from build123d import *

# Parameters (mm, degrees)
BOSS_EXTRUDE1_DEPTH = 64.25


with BuildPart() as part:
    # Sketch1 → Boss-Extrude1 (new body, symmetric)
    with BuildSketch(Plane(origin=(0, 0, 0), x_dir=(1, 0, 0), z_dir=(0, 1, 0))):
        with BuildLine():
            Line((-27.932619, -6.859853), (-27.932619, 5.140147))
            ThreePointArc((-27.932619, 5.140147), (-26.761046, 7.968574), (-23.932619, 9.140147))
            Line((-23.932619, 9.140147), (-11.932619, 9.140147))
            Line((-11.932619, 9.140147), (-11.932619, 4.640147))
            Line((-11.932619, 4.640147), (-19.182619, 4.640147))
            Line((-19.182619, 4.640147), (-19.182619, 3.140147))
            Line((-19.182619, 3.140147), (-12.932619, -3.109853))
            Line((-12.932619, -3.109853), (-7.932619, -3.109853))
            Line((-7.932619, -3.109853), (-2.932619, -3.109853))
            Line((-2.932619, -3.109853), (3.317381, 3.140147))
            Line((3.317381, 3.140147), (3.317381, 4.640147))
            Line((3.317381, 4.640147), (-3.932619, 4.640147))
            Line((-3.932619, 4.640147), (-3.932619, 9.140147))
            Line((-3.932619, 9.140147), (8.067381, 9.140147))
            ThreePointArc((8.067381, 9.140147), (10.895808, 7.968574), (12.067381, 5.140147))
            Line((12.067381, 5.140147), (12.067381, -6.859853))
            Line((12.067381, -6.859853), (7.567381, -6.859853))
            Line((7.567381, -6.859853), (7.567381, 0.390147))
            Line((7.567381, 0.390147), (6.067381, 0.390147))
            Line((6.067381, 0.390147), (-0.182619, -5.859853))
            Line((-0.182619, -5.859853), (-0.182619, -10.859853))
            Line((-0.182619, -10.859853), (-0.182619, -15.859853))
            Line((-0.182619, -15.859853), (6.067381, -22.109853))
            Line((6.067381, -22.109853), (7.567381, -22.109853))
            Line((7.567381, -22.109853), (7.567381, -14.859853))
            Line((7.567381, -14.859853), (12.067381, -14.859853))
            Line((12.067381, -14.859853), (12.067381, -26.859853))
            ThreePointArc((12.067381, -26.859853), (10.895808, -29.68828), (8.067381, -30.859853))
            Line((8.067381, -30.859853), (-3.932619, -30.859853))
            Line((-3.932619, -30.859853), (-3.932619, -26.359853))
            Line((-3.932619, -26.359853), (3.317381, -26.359853))
            Line((3.317381, -26.359853), (3.317381, -24.859853))
            Line((3.317381, -24.859853), (-2.932619, -18.609853))
            Line((-2.932619, -18.609853), (-7.932619, -18.609853))
            Line((-7.932619, -18.609853), (-12.932619, -18.609853))
            Line((-12.932619, -18.609853), (-19.182619, -24.859853))
            Line((-19.182619, -24.859853), (-19.182619, -26.359853))
            Line((-19.182619, -26.359853), (-11.932619, -26.359853))
            Line((-11.932619, -26.359853), (-11.932619, -30.859853))
            Line((-11.932619, -30.859853), (-23.932619, -30.859853))
            ThreePointArc((-23.932619, -30.859853), (-26.761046, -29.68828), (-27.932619, -26.859853))
            Line((-27.932619, -26.859853), (-27.932619, -14.859853))
            Line((-27.932619, -14.859853), (-23.432619, -14.859853))
            Line((-23.432619, -14.859853), (-23.432619, -22.109853))
            Line((-23.432619, -22.109853), (-21.932619, -22.109853))
            Line((-21.932619, -22.109853), (-15.682619, -15.859853))
            Line((-15.682619, -15.859853), (-15.682619, -10.859853))
            Line((-15.682619, -10.859853), (-15.682619, -5.859853))
            Line((-15.682619, -5.859853), (-21.932619, 0.390147))
            Line((-21.932619, 0.390147), (-23.432619, 0.390147))
            Line((-23.432619, 0.390147), (-23.432619, -6.859853))
            Line((-23.432619, -6.859853), (-27.932619, -6.859853))
        make_face()
        with BuildLine():
            Line((-25.932619, 2.390147), (-25.932619, 5.140147))
            ThreePointArc((-25.932619, 5.140147), (-25.346832, 6.554361), (-23.932619, 7.140147))
            Line((-23.932619, 7.140147), (-21.182619, 7.140147))
            Line((-21.182619, 7.140147), (-21.182619, 3.097254))
            Line((-21.182619, 3.097254), (-20.734396, 2.649031))
            Line((-20.734396, 2.649031), (-21.441502, 1.941924))
            Line((-21.441502, 1.941924), (-21.889726, 2.390147))
            Line((-21.889726, 2.390147), (-25.932619, 2.390147))
        make_face(mode=Mode.SUBTRACT)
        with BuildLine():
            Line((-20.380842, 0.881264), (-13.682619, -5.816959))
            Line((-13.682619, -5.816959), (-13.682619, -7.955115))
            Line((-13.682619, -7.955115), (-13.182619, -7.955115))
            Line((-13.182619, -7.955115), (-12.002324, -7.955115))
            ThreePointArc((-12.002324, -7.955115), (-11.468153, -7.324319), (-10.837356, -6.790148))
            Line((-10.837356, -6.790148), (-10.837356, -5.609853))
            Line((-10.837356, -5.609853), (-10.837356, -5.109853))
            Line((-10.837356, -5.109853), (-12.975512, -5.109853))
            Line((-12.975512, -5.109853), (-19.673735, 1.588371))
            Line((-19.673735, 1.588371), (-20.380842, 0.881264))
        make_face(mode=Mode.SUBTRACT)
        with BuildLine():
            Line((10.067381, 2.390147), (10.067381, 5.140147))
            ThreePointArc((10.067381, 5.140147), (9.481595, 6.554361), (8.067381, 7.140147))
            Line((8.067381, 7.140147), (5.317381, 7.140147))
            Line((5.317381, 7.140147), (5.317381, 3.097254))
            Line((5.317381, 3.097254), (4.869158, 2.649031))
            Line((4.869158, 2.649031), (5.576265, 1.941924))
            Line((5.576265, 1.941924), (6.024488, 2.390147))
            Line((6.024488, 2.390147), (10.067381, 2.390147))
        make_face(mode=Mode.SUBTRACT)
        with BuildLine():
            Line((-2.182619, -5.816959), (-2.182619, -7.955115))
            Line((-2.182619, -7.955115), (-2.682619, -7.955115))
            Line((-2.682619, -7.955115), (-3.862914, -7.955115))
            ThreePointArc((-3.862914, -7.955115), (-4.397085, -7.324319), (-5.027881, -6.790148))
            Line((-5.027881, -6.790148), (-5.027881, -5.609853))
            Line((-5.027881, -5.609853), (-5.027881, -5.109853))
            Line((-5.027881, -5.109853), (-2.889726, -5.109853))
            Line((-2.889726, -5.109853), (3.808498, 1.588371))
            Line((3.808498, 1.588371), (4.515604, 0.881264))
            Line((4.515604, 0.881264), (-2.182619, -5.816959))
        make_face(mode=Mode.SUBTRACT)
        with BuildLine():
            Line((5.317381, -28.859853), (8.067381, -28.859853))
            ThreePointArc((8.067381, -28.859853), (9.481595, -28.274066), (10.067381, -26.859853))
            Line((10.067381, -26.859853), (10.067381, -24.109853))
            Line((10.067381, -24.109853), (6.024488, -24.109853))
            Line((6.024488, -24.109853), (5.576265, -23.661629))
            Line((5.576265, -23.661629), (4.869158, -24.368736))
            Line((4.869158, -24.368736), (5.317381, -24.816959))
            Line((5.317381, -24.816959), (5.317381, -28.859853))
        make_face(mode=Mode.SUBTRACT)
        with BuildLine():
            Line((-2.889726, -16.609853), (-5.027881, -16.609853))
            Line((-5.027881, -16.609853), (-5.027881, -16.109853))
            Line((-5.027881, -16.109853), (-5.027881, -14.929558))
            ThreePointArc((-5.027881, -14.929558), (-4.397085, -14.395387), (-3.862914, -13.76459))
            Line((-3.862914, -13.76459), (-2.682619, -13.76459))
            Line((-2.682619, -13.76459), (-2.182619, -13.76459))
            Line((-2.182619, -13.76459), (-2.182619, -15.902746))
            Line((-2.182619, -15.902746), (4.515604, -22.600969))
            Line((4.515604, -22.600969), (3.808498, -23.308076))
            Line((3.808498, -23.308076), (-2.889726, -16.609853))
        make_face(mode=Mode.SUBTRACT)
        with BuildLine():
            Line((-25.932619, -24.109853), (-25.932619, -26.859853))
            ThreePointArc((-25.932619, -26.859853), (-25.346832, -28.274066), (-23.932619, -28.859853))
            Line((-23.932619, -28.859853), (-21.182619, -28.859853))
            Line((-21.182619, -28.859853), (-21.182619, -24.816959))
            Line((-21.182619, -24.816959), (-20.734396, -24.368736))
            Line((-20.734396, -24.368736), (-21.441502, -23.661629))
            Line((-21.441502, -23.661629), (-21.889726, -24.109853))
            Line((-21.889726, -24.109853), (-25.932619, -24.109853))
        make_face(mode=Mode.SUBTRACT)
        with BuildLine():
            Line((-13.682619, -15.902746), (-13.682619, -13.76459))
            Line((-13.682619, -13.76459), (-13.182619, -13.76459))
            Line((-13.182619, -13.76459), (-12.002324, -13.76459))
            ThreePointArc((-12.002324, -13.76459), (-11.468153, -14.395387), (-10.837356, -14.929558))
            Line((-10.837356, -14.929558), (-10.837356, -16.109853))
            Line((-10.837356, -16.109853), (-10.837356, -16.609853))
            Line((-10.837356, -16.609853), (-12.975512, -16.609853))
            Line((-12.975512, -16.609853), (-19.673735, -23.308076))
            Line((-19.673735, -23.308076), (-20.380842, -22.600969))
            Line((-20.380842, -22.600969), (-13.682619, -15.902746))
        make_face(mode=Mode.SUBTRACT)
        with BuildLine():
            ThreePointArc((-11.332619, -10.859853), (-10.336782, -8.45569), (-7.932619, -7.459853))
            ThreePointArc((-7.932619, -7.459853), (-5.528456, -8.45569), (-4.532619, -10.859853))
            ThreePointArc((-4.532619, -10.859853), (-5.528456, -13.264016), (-7.932619, -14.259853))
            ThreePointArc((-7.932619, -14.259853), (-10.336782, -13.264016), (-11.332619, -10.859853))
        make_face(mode=Mode.SUBTRACT)
    extrude(amount=BOSS_EXTRUDE1_DEPTH, both=True)


solid = part.part
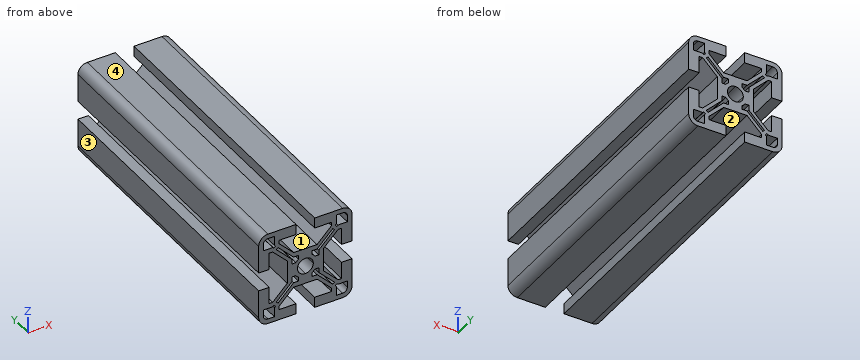
The listing builds one solid part. Answer for the finished solid, in the listing's coordinates (mm). Face numbers are marked on the shaded views. Give positions to 0.01 mm unless a question says otherwise; leave off trailing zeros. Order: outer loops, then holes, each group sorted by start corner. A loop starts at its lowest first (then second) coordinate and runs counter-clockwise, first axis right, second up. Notation, with made-up numbers: (71, 9) - (96, 9) arc R31 cw to (96, 41) - close; hole circle Ø2 at (89.25, 46). An arc over 180 degrees is marked (long way). One line per item, written item: value. Start each with the question number.
1) Find the intervals of material crossed by L1, parallel to Z at x = 7.5, y = 33; L2, parallel to Z at x = 8, y = -4.5; L3, parallel to Z at x = -12, y = 35.5, in increasing order.
2) A cutting plane is placed at B-B on y = 31.5. State how many separate pieces and enclosed holes the cut face has, then the cut area to 3 significant figures.
3) A cutting plane is placed at A-A on x = 1.5. Give the vertices of the cut face in (y, z), then the cut area to 3 significant figures.
4) Given pin 1 Ø1.3 at (y, z) = (-24.5, 29.5) entering from -X, flat-ended and moving along its own axis, determine where the tip first touches the part or whether it passes through.
5) The mould has two halves that part along X. Classify the marked faces 1, 2, 3 and 4: released by +X, released by -X, zero draft, split by the parting line, or undercut.
Answer sheet:
1. L1: z = -9.14 to -7.14, -2.39 to -0.39, 22.11 to 24.11, 28.86 to 30.86
1. L2: z = -9.14 to -7.14, -2.39 to 6.86, 14.86 to 24.11, 28.86 to 30.86
1. L3: z = -9.14 to -4.64, 3.11 to 5.11, 7.95 to 13.77, 16.61 to 18.61, 26.36 to 30.86
2. separate pieces: 1
2. enclosed holes: 9
2. area: 710 mm2
3. outline: (-64.25, -9.14) - (64.25, -9.14) - (64.25, -4.64) - (-64.25, -4.64) - close; (-64.25, -1.32) - (64.25, -1.32) - (64.25, 0.72) - (-64.25, 0.72) - close; (-64.25, 2.13) - (64.25, 2.13) - (64.25, 4.18) - (-64.25, 4.18) - close; (-64.25, 17.54) - (64.25, 17.54) - (64.25, 19.59) - (-64.25, 19.59) - close; (-64.25, 21) - (64.25, 21) - (64.25, 23.04) - (-64.25, 23.04) - close; (-64.25, 26.36) - (64.25, 26.36) - (64.25, 30.86) - (-64.25, 30.86) - close
3. area: 2,210 mm2
4. pin 1: stops at x = -27.4
5. face 1: undercut
5. face 2: undercut
5. face 3: released by -X
5. face 4: zero draft
